```python
from build123d import *

# Parameters (mm, degrees)
SKETCH1_W                                           = 85
SKETCH1_H                                           = 200
BOSS_EXTRUDE1_DEPTH                                 = 5
SKETCH2_3_R                                         = 2.5
LED_THRU_HOLE_DEPTH                                 = 5
F_1_4_40_THREADED_THROUGH_HOLE_REACH                = 193.839
SKETCH3_R                                           = 2.82956
CBORE_FOR_4_BINDING_HEAD_MACHINE_SCREW1_D           = 3.4544
CBORE_FOR_4_BINDING_HEAD_MACHINE_SCREW1_CBORE_D     = 6.74624
CBORE_FOR_4_BINDING_HEAD_MACHINE_SCREW1_CBORE_DEPTH = 1.7272
SKETCH2_7_W                                         = 19.5
SKETCH2_7_H                                         = 11
RS232_FEEDTHRUS_DEPTH                               = 5
ELECTRONICS_START                                   = 3
ELECTRONICS_RECESS_OUTLINE_W                        = 70
ELECTRONICS_RECESS_OUTLINE_H                        = 111.786888031
ELECTRONICS_RECESS_OUTLINE_R                        = 5
ELECTRONICS_RECESS_OUTLINE_W_2                      = 19.5
ELECTRONICS_RECESS_OUTLINE_H_2                      = 11
ELECTRONICS_RECESS_OUTLINE_W_3                      = 8
ELECTRONICS_RECESS_OUTLINE_R_2                      = 2.5
ELECTRONICS_RECESS_DEPTH                            = 2
FILLET4_R                                           = 2
CBORE_FOR_4_BINDING_HEAD_MACHINE_SCREW2_D           = 3.2639
CBORE_FOR_4_BINDING_HEAD_MACHINE_SCREW2_CBORE_D     = 6.74624
CBORE_FOR_4_BINDING_HEAD_MACHINE_SCREW2_CBORE_DEPTH = 1.7272
F_4_40_TAPPED_HOLE1_D                               = 2.2606
F_4_40_TAPPED_HOLE1_DEPTH                           = 7.6
F_4_40_TAPPED_HOLE1_TIP                             = 0.679152758
F_4_40_TAPPED_HOLE3_D                               = 2.2606
SKETCH3_4_R                                         = 7.5
SKETCH3_4_R_2                                       = 2.82956
CUT_EXTRUDE1_DEPTH                                  = 2
SKETCH2_11_R                                        = 5
CUT_EXTRUDE2_DEPTH                                  = 192.838916346


# Read off the part's stored shape, not the designer's step: electronics recess
with BuildPart() as part:
    # Sketch1 → Boss-Extrude1 (new body)
    with BuildSketch(Plane.XY):
        with Locations((-115.863171355, -8.158567775)):
            Rectangle(SKETCH1_W, SKETCH1_H)
    extrude(amount=BOSS_EXTRUDE1_DEPTH)

    # Sketch2<3> (on Front Plane) → LED thru hole (cut)
    with BuildSketch(Plane.XY):
        with Locations((-138.363171355, -78.158567775)):
            Circle(SKETCH2_3_R)
    extrude(amount=LED_THRU_HOLE_DEPTH, mode=Mode.SUBTRACT)

    # Sketch3 → 1/4-40 threaded through hole (cut, up to next)
    with BuildSketch(Plane.XY.offset(5), mode=Mode.PRIVATE) as f_1_4_40_threaded_through_hole_sk1:
        with Locations((-98.363171355, -78.158567775)):
            Circle(SKETCH3_R)
    f_1_4_40_threaded_through_hole_tool1 = extrude(f_1_4_40_threaded_through_hole_sk1.sketch, amount=-F_1_4_40_THREADED_THROUGH_HOLE_REACH, mode=Mode.PRIVATE) & part.part
    add(f_1_4_40_threaded_through_hole_tool1.solids().sort_by_distance((-98.363171, -78.158568, 5))[0], mode=Mode.SUBTRACT)

    # CBORE for #4 Binding Head Machine Screw1 (through all)
    with Locations(Plane(origin=(0, 0, 0), x_dir=(-1, 0, 0), z_dir=(0, 0, -1))):
        with Locations((78.363171355, 56.841432225), (78.363171355, -8.158567775), (78.363171355, -73.158567775)):
            CounterBoreHole(CBORE_FOR_4_BINDING_HEAD_MACHINE_SCREW1_D / 2, CBORE_FOR_4_BINDING_HEAD_MACHINE_SCREW1_CBORE_D / 2, CBORE_FOR_4_BINDING_HEAD_MACHINE_SCREW1_CBORE_DEPTH)

    # Sketch2<7> (on Front Plane) → RS232 feedthrus (cut)
    with BuildSketch(Plane.XY):
        with Locations((-118.613171355, 50.841432225)):
            Rectangle(SKETCH2_7_W, SKETCH2_7_H)
        with Locations((-118.613171355, 25.841432225)):
            Rectangle(SKETCH2_7_W, SKETCH2_7_H)
        with Locations((-118.613171355, 0.841432225)):
            Rectangle(SKETCH2_7_W, SKETCH2_7_H)
    extrude(amount=RS232_FEEDTHRUS_DEPTH, mode=Mode.SUBTRACT)

    # electronics recess outline → electronics recess (cut)
    # profile 1 of 2: a face of its own
    with BuildSketch(Plane.XY.offset(ELECTRONICS_START)):
        with Locations((-123.363171355, 10.44798821)):
            Rectangle(ELECTRONICS_RECESS_OUTLINE_W, ELECTRONICS_RECESS_OUTLINE_H)
        with Locations((-138.363171355, -30.052011791)):
            Circle(ELECTRONICS_RECESS_OUTLINE_R, mode=Mode.SUBTRACT)
        with Locations((-108.363171355, -30.052011791)):
            Circle(ELECTRONICS_RECESS_OUTLINE_R, mode=Mode.SUBTRACT)
        with Locations((-118.613171355, 0.841432225)):
            Rectangle(ELECTRONICS_RECESS_OUTLINE_W_2, ELECTRONICS_RECESS_OUTLINE_H_2, mode=Mode.SUBTRACT)
        with Locations((-118.613171355, 25.841432225)):
            Rectangle(ELECTRONICS_RECESS_OUTLINE_W_2, ELECTRONICS_RECESS_OUTLINE_H_2, mode=Mode.SUBTRACT)
        with Locations((-118.613171355, 50.841432225)):
            Rectangle(ELECTRONICS_RECESS_OUTLINE_W_2, ELECTRONICS_RECESS_OUTLINE_H_2, mode=Mode.SUBTRACT)
    # profile 2 of 2: a face of its own
    with BuildSketch(Plane.XY.offset(ELECTRONICS_START)):
        with Locations((-138.363171355, -78.158567775)):
            Rectangle(ELECTRONICS_RECESS_OUTLINE_W_3, ELECTRONICS_RECESS_OUTLINE_H_2)
        with Locations((-138.363171355, -78.158567775)):
            Circle(ELECTRONICS_RECESS_OUTLINE_R_2, mode=Mode.SUBTRACT)
    extrude(amount=ELECTRONICS_RECESS_DEPTH, mode=Mode.SUBTRACT)

    # Fillet4
    fillet4_edges = [part.edges().sort_by_distance(p)[0] for p in [
        (-134.363171355, -83.658567775, 4),
        (-142.363171355, -83.658567775, 4),
        (-142.363171355, -72.658567775, 4),
        (-134.363171355, -72.658567775, 4),
        (-88.363171355, -45.445455806, 4),
        (-88.363171355, 66.341432225, 4),
        (-128.363171355, 45.341432225, 1.5),
        (-128.363171355, 56.341432225, 1.5),
        (-108.863171355, 56.341432225, 1.5),
        (-108.863171355, 45.341432225, 1.5),
        (-128.363171355, 20.341432225, 1.5),
        (-128.363171355, 31.341432225, 1.5),
        (-108.863171355, 31.341432225, 1.5),
        (-108.863171355, 20.341432225, 1.5),
        (-108.863171355, 6.341432225, 1.5),
        (-108.863171355, -4.658567775, 1.5),
        (-128.363171355, -4.658567775, 1.5),
        (-128.363171355, 6.341432225, 1.5),
    ]]
    fillet(fillet4_edges, radius=FILLET4_R)

    # CBORE for #4 Binding Head Machine Screw2 (through all)
    with Locations(Plane(origin=(0, 0, 0), x_dir=(-1, 0, 0), z_dir=(0, 0, -1))):
        with Locations((143.363171355, 86.841432225), (115.863171355, 86.841432225), (88.363171355, 86.841432225), (88.363171355, -103.158567775), (115.863171355, -103.158567775), (143.363171355, -103.158567775)):
            CounterBoreHole(CBORE_FOR_4_BINDING_HEAD_MACHINE_SCREW2_D / 2, CBORE_FOR_4_BINDING_HEAD_MACHINE_SCREW2_CBORE_D / 2, CBORE_FOR_4_BINDING_HEAD_MACHINE_SCREW2_CBORE_DEPTH)

    # #4-40 Tapped Hole1
    with Locations(Plane.ZY.offset(158.363171355)):
        with Locations((2.5, -58.158567775)):
            Hole(F_4_40_TAPPED_HOLE1_D / 2, depth=F_4_40_TAPPED_HOLE1_DEPTH)
            with Locations((0, 0, -(F_4_40_TAPPED_HOLE1_DEPTH + F_4_40_TAPPED_HOLE1_TIP / 2))):  # 118° drill point
                Cone(0, F_4_40_TAPPED_HOLE1_D / 2, F_4_40_TAPPED_HOLE1_TIP, mode=Mode.SUBTRACT)

    # #4-40 Tapped Hole3 (through all)
    with Locations(Plane.XY.offset(3)):
        with Locations((-131.113171355, 50.841432225), (-106.113171355, 50.841432225), (-106.113171355, 25.841432225), (-131.113171355, 25.841432225), (-131.113171355, 0.841432225), (-106.113171355, 0.841432225)):
            Hole(F_4_40_TAPPED_HOLE3_D / 2)

    # Sketch3<4> → Cut-Extrude1 (cut)
    with BuildSketch(Plane.XY.offset(5)):
        with Locations((-98.363171355, -78.158567775)):
            Circle(SKETCH3_4_R)
        with Locations((-98.363171355, -78.158567775)):
            Circle(SKETCH3_4_R_2, mode=Mode.SUBTRACT)
    extrude(amount=-CUT_EXTRUDE1_DEPTH, mode=Mode.SUBTRACT)

    # Sketch2<11> (on Front Plane) → Cut-Extrude2 (cut, through all)
    with BuildSketch(Plane.XY):
        with Locations((-138.363171355, -30.052011791)):
            Circle(SKETCH2_11_R)
        with Locations((-108.363171355, -30.052011791)):
            Circle(SKETCH2_11_R)
    extrude(amount=CUT_EXTRUDE2_DEPTH, mode=Mode.SUBTRACT)


solid = part.part
```
Geometry: final body of the model. Coordinates: model frame, mm. A direction names the side the tool comes from. Coordinates: 2 decimals unless noted, no trailing zeros. Order: outer loops, then holes, each group sorted by start corner. A loop starts at its lowest first (then second) coordinate and runs counter-clockwise, first axis right, second up. Notation, with made-up numbers: M -15.5,89.5 L 1.5,89.5 A15 cw 1.5,106.5 Z; hole C 49,84 d4. An arc over 180 degrees is marked long. Answer as CSV lines item,"result".
Q1. Draft query along X for faces 4 (the cylindrical face through (-91.58, -102.15, 0.85)), 5 (the flat face through (-116, -108.159, 2)), 6 (the flat face through (-158.363, -10, 2)). Return one class per face: pulls with the +X half, pulls with the -X half, needs draft (parallel to the pull), parting line crosses it, or undercut.
Answers:
face 4,"undercut"
face 5,"needs draft"
face 6,"pulls with the -X half"
Q2. First-contact query: P1, Ø2, axis at x = -143.5, y = -104.5, coming from the -Z side; P2, Ø0.6, axis at y = 34, z = 4, coming from the -X side; P3, Ø11, axis at x = -88.36, y = -103.16, coming from the -Z side. Flat tips, straight axial feed; report the tip coordinate or a pass-through.
Answers:
P1,"stops at z = 1.73"
P2,"stops at x = -88.36"
P3,"stops at z = 0"
Q3. Section B-B on y = 16. Return the cut outline in (x, z).
Answers:
outline,"M -158.36,0 L -73.36,0 L -73.36,5 L -88.36,5 L -88.36,3 L -158.36,3 Z"
Q4. Line query: probe 1 along Y at (x, z) = (-121.5, 1.35); probe 2 along X at (y, z) = (-75, 4.75); probe 3 along Y at (x, z) = (-81, 1.4). Output: solid intervals per line, ascending. Write a range as [from, to].
Answers:
probe 1,"y = [-108.16, -4.66], [6.34, 20.34], [31.34, 45.34], [56.34, 91.84]"
probe 2,"x = [-158.36, -142.36], [-134.36, -105.17], [-91.56, -73.36]"
probe 3,"y = [-108.16, -75.26], [-71.05, -10.26], [-6.05, 54.74], [58.95, 91.84]"
Q5. Set-up query: faces 1 (the cylindrical face through (-105.856, -77.829, 4.014)), 2 (the cylindrical face through (-81.58, -7.15, 0.85)), 3 (the cylindrical face through (-113.36, -29.83, 1.48)). Return all of +Z, -Z, +X, -X, +Y, -Y with unobstructed straight access to the full face (end or side cutting, diameter ignored); none if empty.
Answers:
face 1,"+Z"
face 2,"-Z"
face 3,"+Z, -Z"
Q6. Section A-A on x = -99. Return the cut outline in (y, z).
Answers:
outline,"M -108.16,0 L -80.92,0 L -80.92,3 L -85.63,3 L -85.63,5 L -108.16,5 Z; M -75.4,0 L 91.84,0 L 91.84,5 L 66.34,5 L 66.34,3 L -45.45,3 L -45.45,5 L -70.69,5 L -70.69,3 L -75.4,3 Z"
